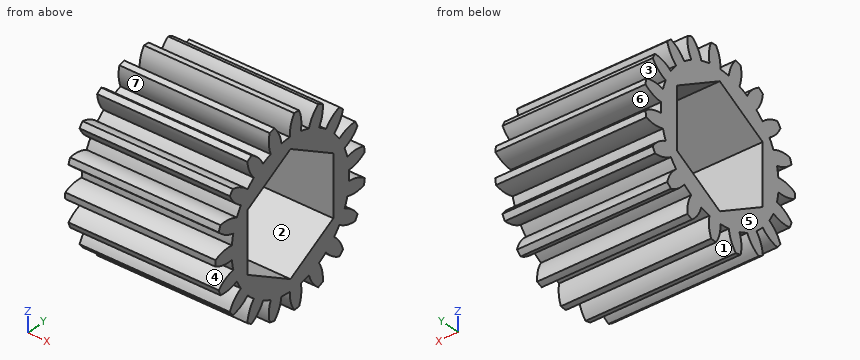
```python
from build123d import *

# Parameters (mm, degrees)
SPUR_START             = -56.943752669
SPUR_GEAR_AI_OUTLINE_R = 4.7625
SPUR_GEAR_AI_DEPTH     = 13.8176
CUT_EXTRUDE1_DEPTH     = 40.482760103


# Read off the part's stored shape, not the designer's step: spur gear_ai
with BuildPart() as part:
    # spur gear_ai outline → spur gear_ai (new body)
    with BuildSketch(Plane.YZ.offset(SPUR_START)):
        with BuildLine():
            ThreePointArc((13.877482254, 21.299310941), (14.013498804, 21.54095532), (14.141401376, 21.786990765))
            ThreePointArc((14.141401376, 21.786990765), (13.511259094, 22.480540591), (12.698675372, 22.947229299))
            ThreePointArc((12.698675372, 22.947229299), (12.866749459, 23.385013416), (13.003007958, 23.833719839))
            ThreePointArc((13.003007958, 23.833719839), (13.930896828, 23.702903551), (14.85415475, 23.863170414))
            ThreePointArc((14.85415475, 23.863170414), (14.904339747, 24.135886336), (14.945424627, 24.410120799))
            ThreePointArc((14.945424627, 24.410120799), (14.124229931, 24.861485317), (13.20414066, 25.039042041))
            ThreePointArc((13.20414066, 25.039042041), (13.220959759, 25.507679374), (13.20414066, 25.976316707))
            ThreePointArc((13.20414066, 25.976316707), (14.124229931, 26.15387343), (14.945424627, 26.605237949))
            ThreePointArc((14.945424627, 26.605237949), (14.904339747, 26.879472412), (14.85415475, 27.152188334))
            ThreePointArc((14.85415475, 27.152188334), (13.930896828, 27.312455197), (13.003007958, 27.181638909))
            ThreePointArc((13.003007958, 27.181638909), (12.866749459, 27.630345332), (12.698675372, 28.068129449))
            ThreePointArc((12.698675372, 28.068129449), (13.511259094, 28.534818157), (14.141401376, 29.228367983))
            ThreePointArc((14.141401376, 29.228367983), (14.013498804, 29.474403428), (13.877482254, 29.716047807))
            ThreePointArc((13.877482254, 29.716047807), (12.952210428, 29.567849612), (12.117073115, 29.142836288))
            ThreePointArc((12.117073115, 29.142836288), (11.84250274, 29.522987496), (11.5413871, 29.882477695))
            ThreePointArc((11.5413871, 29.882477695), (12.158409219, 30.587725425), (12.529213394, 31.448303673))
            ThreePointArc((12.529213394, 31.448303673), (12.328353358, 31.639478342), (12.121244757, 31.82386526))
            ThreePointArc((12.121244757, 31.82386526), (11.294226586, 31.383261581), (10.642340918, 30.710108009))
            ThreePointArc((10.642340918, 30.710108009), (10.259212627, 30.980508721), (9.857685986, 31.222748662))
            ThreePointArc((9.857685986, 31.222748662), (10.212282581, 32.09013088), (10.283566263, 33.024480543))
            ThreePointArc((10.283566263, 33.024480543), (10.031515064, 33.140077693), (9.775757844, 33.247225967))
            ThreePointArc((9.775757844, 33.247225967), (9.13661358, 32.561963049), (8.738621482, 31.713615864))
            ThreePointArc((8.738621482, 31.713615864), (8.288453171, 31.844963967), (7.830027171, 31.943703192))
            ThreePointArc((7.830027171, 31.943703192), (7.883772199, 32.879225575), (7.647810695, 33.78609537))
            ThreePointArc((7.647810695, 33.78609537), (7.371881992, 33.813588258), (7.095191416, 33.831886709))
            ThreePointArc((7.095191416, 33.831886709), (6.713182256, 32.976223424), (6.612212349, 32.044614206))
            ThreePointArc((6.612212349, 32.044614206), (6.14378674, 32.022676095), (5.678138951, 31.967214677))
            ThreePointArc((5.678138951, 31.967214677), (5.425208304, 32.869498859), (4.907571703, 33.650615372))
            ThreePointArc((4.907571703, 33.650615372), (4.637666652, 33.587024715), (4.370026438, 33.514490423))
            ThreePointArc((4.370026438, 33.514490423), (4.286549003, 32.581151163), (4.493542942, 31.667234227))
            ThreePointArc((4.493542942, 31.667234227), (4.057621217, 31.494387237), (3.635211803, 31.290735282))
            ThreePointArc((3.635211803, 31.290735282), (3.103014441, 32.062004771), (2.359796702, 32.632721907))
            ThreePointArc((2.359796702, 32.632721907), (2.125163704, 32.484938741), (1.895576821, 32.329431921))
            ThreePointArc((1.895576821, 32.329431921), (2.119677185, 31.419558478), (2.612203966, 30.622370905))
            ThreePointArc((2.612203966, 30.622370905), (2.256025009, 30.317345688), (1.922628583, 29.987572046))
            ThreePointArc((1.922628583, 29.987572046), (1.168836349, 30.544247826), (0.280576646, 30.842719527))
            ThreePointArc((0.280576646, 30.842719527), (0.106641826, 30.626758451), (-0.060012425, 30.405130681))
            ThreePointArc((-0.060012425, 30.405130681), (0.447380989, 29.61732196), (1.172067692, 29.023251392))
            ThreePointArc((1.172067692, 29.023251392), (0.934229019, 28.619102165), (0.725974258, 28.198942925))
            ThreePointArc((0.725974258, 28.198942925), (-0.167727764, 28.480700538), (-1.10477271, 28.474582766))
            ThreePointArc((-1.10477271, 28.474582766), (-1.199160815, 28.213846513), (-1.284822859, 27.950114599))
            ThreePointArc((-1.284822859, 27.950114599), (-0.549120347, 27.369741899), (0.32919523, 27.043165102))
            ThreePointArc((0.32919523, 27.043165102), (0.235470351, 26.583687704), (0.17492489, 26.11867364))
            ThreePointArc((0.17492489, 26.11867364), (-0.761840439, 26.094980276), (-1.646127267, 25.784935985))
            ThreePointArc((-1.646127267, 25.784935985), (-1.650740241, 25.507679374), (-1.646127267, 25.230422763))
            ThreePointArc((-1.646127267, 25.230422763), (-0.761840439, 24.920378472), (0.17492489, 24.896685107))
            ThreePointArc((0.17492489, 24.896685107), (0.235470351, 24.431671044), (0.32919523, 23.972193646))
            ThreePointArc((0.32919523, 23.972193646), (-0.549120347, 23.645616848), (-1.284822859, 23.065244149))
            ThreePointArc((-1.284822859, 23.065244149), (-1.199160815, 22.801512235), (-1.10477271, 22.540775982))
            ThreePointArc((-1.10477271, 22.540775982), (-0.167727765, 22.53465821), (0.725974258, 22.816415822))
            ThreePointArc((0.725974258, 22.816415822), (0.934229019, 22.396256583), (1.172067692, 21.992107356))
            ThreePointArc((1.172067692, 21.992107356), (0.447380989, 21.398036788), (-0.060012425, 20.610228067))
            ThreePointArc((-0.060012425, 20.610228067), (0.106641826, 20.388600297), (0.280576646, 20.17263922))
            ThreePointArc((0.280576646, 20.17263922), (1.168836349, 20.471110922), (1.922628583, 21.027786702))
            ThreePointArc((1.922628583, 21.027786702), (2.256025009, 20.69801306), (2.612203966, 20.392987843))
            ThreePointArc((2.612203966, 20.392987843), (2.119677185, 19.59580027), (1.895576821, 18.685926827))
            ThreePointArc((1.895576821, 18.685926827), (2.125163704, 18.530420007), (2.359796702, 18.382636841))
            ThreePointArc((2.359796702, 18.382636841), (3.103014441, 18.953353977), (3.635211803, 19.724623466))
            ThreePointArc((3.635211803, 19.724623466), (4.057621217, 19.520971511), (4.493542942, 19.348124521))
            ThreePointArc((4.493542942, 19.348124521), (4.286549003, 18.434207585), (4.370026438, 17.500868325))
            ThreePointArc((4.370026438, 17.500868325), (4.637666652, 17.428334032), (4.907571703, 17.364743376))
            ThreePointArc((4.907571703, 17.364743376), (5.425208304, 18.145859889), (5.678138951, 19.048144071))
            ThreePointArc((5.678138951, 19.048144071), (6.14378674, 18.992682653), (6.612212349, 18.970744542))
            ThreePointArc((6.612212349, 18.970744542), (6.713182256, 18.039135324), (7.095191416, 17.183472039))
            ThreePointArc((7.095191416, 17.183472039), (7.371881992, 17.20177049), (7.647810695, 17.229263378))
            ThreePointArc((7.647810695, 17.229263378), (7.883772199, 18.136133173), (7.830027171, 19.071655555))
            ThreePointArc((7.830027171, 19.071655555), (8.288453171, 19.17039478), (8.738621482, 19.301742883))
            ThreePointArc((8.738621482, 19.301742883), (9.13661358, 18.453395698), (9.775757844, 17.768132781))
            ThreePointArc((9.775757844, 17.768132781), (10.031515064, 17.875281055), (10.283566263, 17.990878205))
            ThreePointArc((10.283566263, 17.990878205), (10.212282581, 18.925227868), (9.857685986, 19.792610086))
            ThreePointArc((9.857685986, 19.792610086), (10.259212627, 20.034850026), (10.642340918, 20.305250738))
            ThreePointArc((10.642340918, 20.305250738), (11.294226586, 19.632097166), (12.121244757, 19.191493488))
            ThreePointArc((12.121244757, 19.191493488), (12.328353358, 19.375880406), (12.529213394, 19.567055074))
            ThreePointArc((12.529213394, 19.567055074), (12.158409219, 20.427633322), (11.5413871, 21.132881053))
            ThreePointArc((11.5413871, 21.132881053), (11.84250274, 21.492371252), (12.117073115, 21.87252246))
            ThreePointArc((12.117073115, 21.87252246), (12.952210428, 21.447509136), (13.877482254, 21.299310941))
        make_face()
        with Locations((6.683634759, 25.507679374)):
            Circle(SPUR_GEAR_AI_OUTLINE_R, mode=Mode.SUBTRACT)
    extrude(amount=SPUR_GEAR_AI_DEPTH)

    # Sketch1 → Cut-Extrude1 (cut, through all)
    with BuildSketch(Plane(origin=(-43.126152669, 0, 0), x_dir=(0, 0, -1), z_dir=(1, 0, 0))):
        Polygon((-22.758048717, 11.446134759), (-28.257310031, 11.446134759), (-31.006940688, 6.683634759), (-28.257310031, 1.921134759), (-22.758048717, 1.921134759), (-20.00841806, 6.683634759), align=None)
    extrude(amount=-CUT_EXTRUDE1_DEPTH, mode=Mode.SUBTRACT)


solid = part.part
```
Verification items for the finished model (mm, model axes). Face numbers are marked on the shaded views. A direction names the side the tool comes from. Give positions to 0.01 mm unless a question says otherwise; leave off trailing zeros. Loops run counter-clockwise (first coordinate to the right, second up) from the corner with the lowest first, then second, coordinate; pieces in that order, holes last. Notation, with made-up numbers: M 77.5,89 L 104.5,89 A20 cw 104.5,116 Z; hole C 85,51.5 d4. An arc over 180 degrees is marked long. Return JSON: item names as keys, results as strings.
1) Gauge pin test, flat ends, axial feed: P1, Ø8, axis at x = -53, z = 31, coming from the +Y side; P2, Ø3, axis at x = -55, z = 22, coming from the -Y side. Record the tip position at first contact, or that the pin passes through.
Findings:
{"P1": "stops at y = 14.88", "P2": "stops at y = -1.28"}
2) Material ranges on L1, parallel to Z at x = -46, y = -0.25; L2, parallel to Y at x = -44.5, z = 31.5; L3, parallel to Z at x = -55.5, y = 2.25, recorded low to high. Write a range as [from, to].
Findings:
{"L1": "z = [22.52, 23.79], [24.87, 26.14], [27.22, 28.49]", "L2": "y = [2.09, 3.52], [4.07, 10.01], [11.46, 12.48]", "L3": "z = [18.45, 19.87], [20.7, 22.57], [28.45, 30.31], [31.15, 32.56]"}
3) Mould release check, pull along Y, two halves, no side actions. Record for the marked faces 5, 6 and 7: released by +Y, released by -Y, zero draft, split by the parting line, or undercut.
Findings:
{"face 5": "zero draft", "face 6": "released by +Y", "face 7": "undercut"}
4) Section check A-A, the plane y = 4. Enter the section's corners in (x, z), and give its area (3 significant figures).
Findings:
{"outline": "M -56.94,19.55 L -43.13,19.55 L -43.13,21.56 L -56.94,21.56 Z; M -56.94,29.46 L -43.13,29.46 L -43.13,31.47 L -56.94,31.47 Z", "area": "55.6 mm2"}
5) Tool access check on the marked faces 1, 2, 3 and 4. Record the directions out of +Z, -Z, +X, -X, +Y, -Y that give a thin tool (end or side, any length) a straight path to the whole face; none if there is none.
Findings:
{"face 1": "-Z, +X, -X", "face 2": "+X, -X", "face 3": "+X, -X, +Y", "face 4": "+X, -X, -Y"}
6) Section check B-B, the plane y = 9.25. Enter the section's corners in (x, z).
Findings:
{"outline": "M -56.94,18.3 L -43.13,18.3 L -43.13,21.49 L -56.94,21.49 Z; M -56.94,29.53 L -43.13,29.53 L -43.13,32.72 L -56.94,32.72 Z"}
